The figure shows three views and two pictorial views of one solid part (mm, origin at its lowest corner). Answer the questions. Give positions to 0.01 mm unless a question says otherwise; leave off trailing zeros. Write each loop counter-clockwise with the first axis right and the second up, starting at its lowest first coordinate (ties: lowest second). Pieces come first, ordered by that corner, then holes. Notation, with made-up numbers: (-26, 18.25) - (-11, 18.25) arc R21 ccw to (-11, 53.25) - close; hole circle Ø9 at (54.25, 18.5). An arc over 180 degrees is marked (long way). Use a Markdown table: item, result. Add a question column.
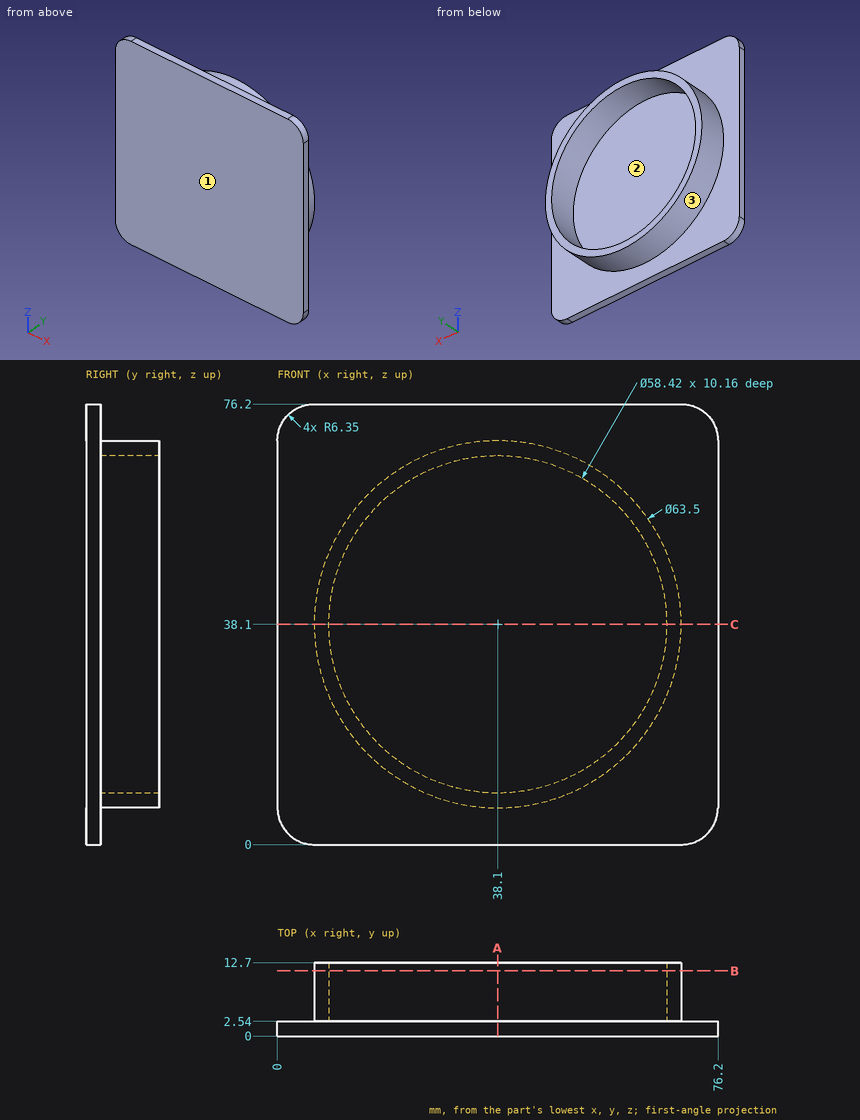
1. Given P1, Ø1.5, axis at y = 9, z = 66, coming from the +X side; P2, Ø1.5, axis at y = 6.5, z = 23, coming from the -X side; P3, Ø2, axis at x = 57.5, y = 10.5, coming from the +Z side, each flat-ended and moving along its own axis, determine where each tip first touches the part or whether it passes through.
2. Consider L1, parallel to X at y = 7, z = 38.1; L2, parallel to Y at x = 72, z = 18.5. Determine where each line is inside the solid, lowest interval first. Write a range as [from, to].
3. For a pull along Z with two mould halves and no side action, classify the marked faces 1, 2 and 3 as released by +Z, released by -Z, zero draft, split by the parting line, or undercut.
4. The part is cut by section B-B (y = 11.25). Give the vertices of the cut face in (x, z).
5. The part is cut by section A-A (x = 38.1). Give the vertices of the cut face in (y, z), and give its area (3 significant figures).
6. The part is cut by section C-C (z = 38.1). Give the vertices of the cut face in (x, y).
Check values:
| question | item | result |
|---|---|---|
| 1 | P1 | stops at x = 54.56 |
| 1 | P2 | stops at x = 9.78 |
| 1 | P3 | stops at z = 63.97 |
| 2 | L1 | x = [6.35, 8.89], [67.31, 69.85] |
| 2 | L2 | y = [0, 2.54] |
| 3 | face 1 | zero draft |
| 3 | face 2 | undercut |
| 3 | face 3 | split by the parting line |
| 4 | outline | circle Ø63.5 at (38.1, 38.1); hole circle Ø58.42 at (38.1, 38.1) |
| 5 | outline | (0, 0) - (2.54, 0) - (2.54, 6.35) - (12.7, 6.35) - (12.7, 8.89) - (2.54, 8.89) - (2.54, 67.31) - (12.7, 67.31) - (12.7, 69.85) - (2.54, 69.85) - (2.54, 76.2) - (0, 76.2) - close |
| 5 | area | 245 mm2 |
| 6 | outline | (0, 0) - (76.2, 0) - (76.2, 2.54) - (69.85, 2.54) - (69.85, 12.7) - (67.31, 12.7) - (67.31, 2.54) - (8.89, 2.54) - (8.89, 12.7) - (6.35, 12.7) - (6.35, 2.54) - (0, 2.54) - close |
